from build123d import *

# Parameters (mm, degrees)
F1_DEPTH = 1.5
F2_R     = 10
F6_DEPTH = 8
F7_DEPTH = 1
F8_W     = 80
F8_H     = 16
F9_DEPTH = 1


with BuildPart() as f1:
    # F0 (on Top) → F1 (new body)
    with BuildSketch(Plane.XY):
        Polygon((40, 0), (-40, 0), (-40, -8), (-75.5, -8), (-75.5, -101), (75.5, -101), (75.5, -8), (40, -8), align=None)
    extrude(amount=F1_DEPTH)

    # F2
    f2_edges = [f1.edges().sort_by_distance(p)[0] for p in [
        (-75.5, -8, 0.75),
        (-75.5, -101, 0.75),
        (75.5, -101, 0.75),
        (75.5, -8, 0.75),
    ]]
    fillet(f2_edges, radius=F2_R)

    # F3: F1 across face


with BuildPart() as f1_1:
    add(f1.part)
    add(f1.part.mirror(Plane(origin=(0, 0, 0.75), x_dir=(-1, 0, 0), z_dir=(0, 1, 0))))

    # F5 (on face) → F6 (join)
    with BuildSketch(Plane.XY.offset(1.5)):
        with BuildLine():
            Line((65.5, -11.3), (40, -11.3))
            Line((40, -11.3), (-40, -11.3))
            Line((-40, -11.3), (-65.5, -11.3))
            ThreePointArc((-65.5, -11.3), (-70.2376154339, -13.2623845661), (-72.2, -18))
            Line((-72.2, -18), (-72.2, -91))
            ThreePointArc((-72.2, -91), (-70.2376154339, -95.7376154339), (-65.5, -97.7))
            Line((-65.5, -97.7), (65.5, -97.7))
            ThreePointArc((65.5, -97.7), (70.2376154339, -95.7376154339), (72.2, -91))
            Line((72.2, -91), (72.2, -18))
            ThreePointArc((72.2, -18), (70.2376154339, -13.2623845661), (65.5, -11.3))
        make_face()
        with BuildLine():
            Line((-70.6, -91), (-70.6, -18))
            ThreePointArc((-70.6, -18), (-69.1062445841, -14.3937554159), (-65.5, -12.9))
            Line((-65.5, -12.9), (-40, -12.9))
            Line((-40, -12.9), (40, -12.9))
            Line((40, -12.9), (65.5, -12.9))
            ThreePointArc((65.5, -12.9), (69.1062445841, -14.3937554159), (70.6, -18))
            Line((70.6, -18), (70.6, -91))
            ThreePointArc((70.6, -91), (69.1062445841, -94.6062445841), (65.5, -96.1))
            Line((65.5, -96.1), (-65.5, -96.1))
            ThreePointArc((-65.5, -96.1), (-69.1062445841, -94.6062445841), (-70.6, -91))
        make_face(mode=Mode.SUBTRACT)
        with BuildLine():
            ThreePointArc((-73.6, 18), (-71.2275649276, 12.2724350724), (-65.5, 9.9))
            Line((-65.5, 9.9), (-40, 9.9))
            Line((-40, 9.9), (40, 9.9))
            Line((40, 9.9), (65.5, 9.9))
            ThreePointArc((65.5, 9.9), (71.2275649276, 12.2724350724), (73.6, 18))
            Line((73.6, 18), (73.6, 91))
            ThreePointArc((73.6, 91), (71.2275649276, 96.7275649276), (65.5, 99.1))
            Line((65.5, 99.1), (-65.5, 99.1))
            ThreePointArc((-65.5, 99.1), (-71.2275649276, 96.7275649276), (-73.6, 91))
            Line((-73.6, 91), (-73.6, 18))
        make_face()
        with BuildLine():
            Line((-72, 18), (-72, 91))
            ThreePointArc((-72, 91), (-70.0961940777, 95.5961940777), (-65.5, 97.5))
            Line((-65.5, 97.5), (65.5, 97.5))
            ThreePointArc((65.5, 97.5), (70.0961940777, 95.5961940777), (72, 91))
            Line((72, 91), (72, 18))
            ThreePointArc((72, 18), (70.0961940777, 13.4038059223), (65.5, 11.5))
            Line((65.5, 11.5), (40, 11.5))
            Line((40, 11.5), (-40, 11.5))
            Line((-40, 11.5), (-65.5, 11.5))
            ThreePointArc((-65.5, 11.5), (-70.0961940777, 13.4038059223), (-72, 18))
        make_face(mode=Mode.SUBTRACT)
    extrude(amount=F6_DEPTH)

    # F7 (add): a face of the model
    f7_faces = [f1_1.faces().sort_by_distance(p)[0] for p in [
        (0, -11.4682745376, 9.5),
    ]]
    extrude(f7_faces, amount=F7_DEPTH)

    # F8 (on face) → F9 (cut, through all)
    with BuildSketch(Plane.XY.offset(1.5)):
        with BuildLine():
            Line((65.5, 97.5), (-65.5, 97.5))
            ThreePointArc((-65.5, 97.5), (-70.0961940777, 95.5961940777), (-72, 91))
            Line((-72, 91), (-72, 18))
            ThreePointArc((-72, 18), (-70.0961940777, 13.4038059223), (-65.5, 11.5))
            Line((-65.5, 11.5), (65.5, 11.5))
            ThreePointArc((65.5, 11.5), (70.0961940777, 13.4038059223), (72, 18))
            Line((72, 18), (72, 91))
            ThreePointArc((72, 91), (70.0961940777, 95.5961940777), (65.5, 97.5))
        make_face()
        Rectangle(F8_W, F8_H)
        with BuildLine():
            Line((70.6, -91), (70.6, -18))
            ThreePointArc((70.6, -18), (69.1062445841, -14.3937554159), (65.5, -12.9))
            Line((65.5, -12.9), (-65.5, -12.9))
            ThreePointArc((-65.5, -12.9), (-69.1062445841, -14.3937554159), (-70.6, -18))
            Line((-70.6, -18), (-70.6, -91))
            ThreePointArc((-70.6, -91), (-69.1062445841, -94.6062445841), (-65.5, -96.1))
            Line((-65.5, -96.1), (65.5, -96.1))
            ThreePointArc((65.5, -96.1), (69.1062445841, -94.6062445841), (70.6, -91))
        make_face()
    extrude(amount=-F9_DEPTH, mode=Mode.SUBTRACT)


solid = f1_1.part
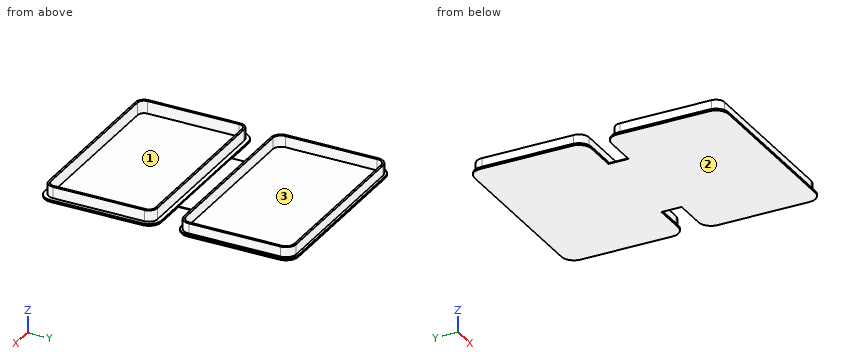
Input: part model. Units: mm. Frame: model coordinates. Face numbers are marked on the shaded views. Round coordinates to 2 decimals unless told otherwise and drop trailing zeros. Loops run counter-clockwise (first coordinate to the right, second up) from the corner with the lowest first, then second, coordinate; pieces in that order, holes last. Notation, with made-up numbers: M 55,70 L 104,70 A28 cw 104,104 Z; hole C -37.5,66 d1. An arc over 180 degrees is marked long. Answer as CSV lines item,"result". Start each with the question number.
(1) Section C-C, the plane x = 9. Output: boundary loops of the cut face in (y, z).
(2) Section A-A, the plane z = 7. State how many separate pieces and enclosed holes the cut face has, plus the area to 3 significant figures.
(3) First-contact query: pin 1 (3 mm diameter, centred on x = -42.5, y = 73.5, fed in from -Z); pin 2 (3 mm diameter, centred on x = -56, z = 6, fed in from +Y); pin 3 (4 mm diameter, centred on y = 12, z = 2, fed in from -X); pin 4 (5 mm diameter, centred on x = 25, z = 6.5, fed in from -Y). Flat tips, straight axial feed; report the tip coordinate or a pass-through.
(4) Section D-D, the plane y = -76. Output: boundary loops of the cut face in (x, z).
(5) Section B-B, the plane y = 73. Output: boundary loops of the cut face in (x, z).
(6) Line query: line 1 (Y direction, x = 7, z = 4.25); line 2 (X direction, y = -31, z = 5); line 3 (Y direction, x = 69, z = 3). Output: solid intervals per line, ascending. Write a range as [from, to].
(7) Draft query along X for the marked faces 1, 2 and 3. Return one class per face: released by +X, released by -X, zero draft, split by the parting line, or undercut.
Values found:
1,outline,"M -101,0 L 101,0 L 101,1.5 L 99.1,1.5 L 99.1,9.5 L 97.5,9.5 L 97.5,0.5 L 11.5,0.5 L 11.5,9.5 L 9.9,9.5 L 9.9,1.5 L 8,1.5 L 8,0.5 L -8,0.5 L -8,1.5 L -11.3,1.5 L -11.3,10.5 L -12.9,10.5 L -12.9,0.5 L -96.1,0.5 L -96.1,10.5 L -97.7,10.5 L -97.7,1.5 L -101,1.5 Z"
2,separate pieces,"2"
2,enclosed holes,"2"
2,area,"1,440 mm²"
3,pin 1,"stops at z = 0"
3,pin 2,"stops at y = 99.1"
3,pin 3,"stops at x = -74.64"
3,pin 4,"stops at y = -97.7"
4,outline,"M -75.5,0 L 75.5,0 L 75.5,1.5 L 72.2,1.5 L 72.2,10.5 L 70.6,10.5 L 70.6,0.5 L -70.6,0.5 L -70.6,10.5 L -72.2,10.5 L -72.2,1.5 L -75.5,1.5 Z"
5,outline,"M -75.5,0 L 75.5,0 L 75.5,1.5 L 73.6,1.5 L 73.6,9.5 L 72,9.5 L 72,0.5 L -72,0.5 L -72,9.5 L -73.6,9.5 L -73.6,1.5 L -75.5,1.5 Z"
6,line 1,"y = [-97.7, -96.1], [-12.9, -11.3], [9.9, 11.5], [97.5, 99.1]"
6,line 2,"x = [-72.2, -70.6], [70.6, 72.2]"
6,line 3,"y = [-96.71, -94.71], [-14.29, -12.29], [10.7, 12.52], [96.48, 98.3]"
7,face 1,"undercut"
7,face 2,"zero draft"
7,face 3,"undercut"
